The listing builds one solid part. Answer for the finished solid, in the listing's coordinates (mm). Round coordinates to 2 decimals unless told otherwise and drop trailing zeros. Write each loop counter-clockwise with the first axis right and the second up, starting at its lowest first coordinate (ties: lowest second). Pieces come first, ordered by that corner, then holes.
Item 1: Find section D-D on z = 2.65. Give the number of separate pieces and of enclosed holes in the cut face, then the cut area to 3 significant figures.
Item 2: Find section B-B on y = -38.5. Give the vertices of the cut face in (x, z), then the cut area to 3 significant figures.
Item 3: Find the intervals of material crossed by probe 1 along X at (y, z) = (-36, 3.85); probe 2 along X at (y, z) = (-26.5, 2.6); probe 3 along Y at (x, z) = (-38, 1.6), in increasing order.
Item 4: Find section A-A on x = -35. Give the vertices of the cut face in (y, z).
Item 5: Each of these flat-tipped pins is pushed along its axis until it touches: pin 1 (1.5 mm diameter, centred on y = -29.5, z = 1.5, fed in from -X); pin 2 (1.5 mm diameter, centred on y = -28.5, z = 1.5, fed in from +X); pin 3 (2.5 mm diameter, centred on x = -78.5, z = 1.5, fed in from +Y). Where does it stop, or does it pass through?
Item 6: Find section C-C on x = 6. Give the vertices of the cut face in (y, z), then the cut area to 3 significant figures.
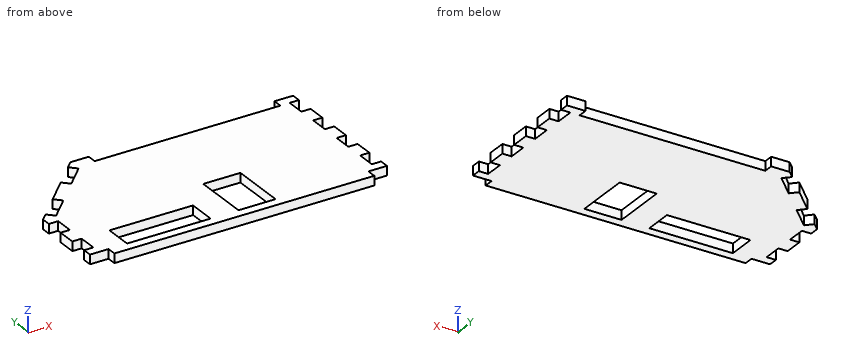
```python
from build123d import *

# Parameters (mm, degrees)
BOSS_EXTRU_1_DEPTH      = 5
ESQUISSE2_W             = 5
ESQUISSE2_H             = 10
ENL_V_MAT_EXTRU_1_DEPTH = 10
ENL_V_MAT_EXTRU_2_DEPTH = 10
ESQUISSE4_W             = 45
ESQUISSE4_H             = 15
ESQUISSE4_W_2           = 20
ESQUISSE4_H_2           = 30
ENL_V_MAT_EXTRU_3_DEPTH = 10


with BuildPart() as part:
    # Esquisse1 → Boss.-Extru.1 (new body)
    with BuildSketch(Plane.XY):
        Polygon((-80, 0), (-40, 40), (-30, 40), (-30, 35), (70, 35), (70, 40), (80, 40), (80, -40), (70, -40), (70, -45), (-70, -45), (-70, -40), (-80, -40), (-80, -35), (-75, -35), (-75, -25), (-80, -25), (-80, -15), (-75, -15), (-75, -5), (-80, -5), align=None)
    extrude(amount=BOSS_EXTRU_1_DEPTH)

    # Esquisse2 → Enlèv. mat.-Extru.1 (cut)
    with BuildSketch(Plane.XY.offset(5)):
        with Locations((77.5, -30)):
            Rectangle(ESQUISSE2_W, ESQUISSE2_H)
        with Locations((77.5, -10)):
            Rectangle(ESQUISSE2_W, ESQUISSE2_H)
        with Locations((77.5, 10)):
            Rectangle(ESQUISSE2_W, ESQUISSE2_H)
        with Locations((77.5, 30)):
            Rectangle(ESQUISSE2_W, ESQUISSE2_H)
    extrude(amount=-ENL_V_MAT_EXTRU_1_DEPTH, mode=Mode.SUBTRACT)

    # Esquisse3 → Enlèv. mat.-Extru.2 (cut)
    with BuildSketch(Plane.XY.offset(5)):
        Polygon((-43.535533906, 36.464466094), (-54.142135624, 25.857864376), (-50.606601718, 22.32233047), (-40, 32.928932188), align=None)
        Polygon((-65.857864376, 14.142135624), (-76.464466094, 3.535533906), (-72.928932188, 0), (-62.32233047, 10.606601718), align=None)
    extrude(amount=-ENL_V_MAT_EXTRU_2_DEPTH, mode=Mode.SUBTRACT)

    # Esquisse4 → Enlèv. mat.-Extru.3 (cut)
    with BuildSketch(Plane.XY.offset(5)):
        with Locations((-37.5, -32.5)):
            Rectangle(ESQUISSE4_W, ESQUISSE4_H)
        with Locations((10, -25)):
            Rectangle(ESQUISSE4_W_2, ESQUISSE4_H_2)
    extrude(amount=-ENL_V_MAT_EXTRU_3_DEPTH, mode=Mode.SUBTRACT)


solid = part.part
```
Check values:
1. separate pieces: 1
1. enclosed holes: 2
1. area: 10,500 mm2
2. outline: (-80, 0) - (-60, 0) - (-60, 5) - (-80, 5) - close; (-15, 0) - (0, 0) - (0, 5) - (-15, 5) - close; (20, 0) - (80, 0) - (80, 5) - (20, 5) - close
2. area: 475 mm2
3. probe 1: x = -80 to -60, -15 to 0, 20 to 80
3. probe 2: x = -75 to -60, -15 to 0, 20 to 75
3. probe 3: y = -45 to -40, -25 to 40
4. outline: (-45, 0) - (-40, 0) - (-40, 5) - (-45, 5) - close; (-25, 0) - (40, 0) - (40, 5) - (-25, 5) - close
5. pin 1: stops at x = -75
5. pin 2: stops at x = 75
5. pin 3: stops at y = 2.75
6. outline: (-45, 0) - (-40, 0) - (-40, 5) - (-45, 5) - close; (-10, 0) - (35, 0) - (35, 5) - (-10, 5) - close
6. area: 250 mm2
